Verification items for the finished model (mm, model axes). Face numbers are marked on the shaded views. A direction names the side the tool comes from. Round coordinates to 2 decimals unless told otherwise and drop trailing zeros. Write each loop counter-clockwise with the first axis right and the second up, starting at its lowest first coordinate (ties: lowest second). Pieces come first, ordered by that corner, then holes.
Autodesk Inventor part; units mm, degrees
ref_plane "YZ Plane" through (0, 0, 0) normal (1, 0, 0) x (0, 1, 0)
ref_plane "XZ Plane" through (0, 0, 0) normal (0, 1, 0) x (-1, 0, 0)
ref_plane "XY Plane" through (0, 0, 0) normal (0, 0, 1) x (1, 0, 0)
sketch "Block1" plane through (0, 0, 0) normal (0, 0, 1) x (1, 0, 0)
  circle A0 centre (74.029, 24.2723) radius 1
  line L0 (49.279, 30.4723) -> (71.779, 30.4723)
  line L1 (71.779, 30.4723) -> (71.779, 18.0723)
  line L2 (71.779, 18.0723) -> (49.279, 18.0723)
  line L3 (49.279, 18.0723) -> (49.279, 30.4723)
  line L4 (49.279, 30.4723) -> (44.779, 30.4723)
  line L5 (44.779, 30.4723) -> (44.779, 18.0723)
  line L6 (44.779, 18.0723) -> (49.279, 18.0723)
  line L7 (49.279, 18.0723) -> (49.279, 30.4723)
  line L8 (71.779, 30.4723) -> (76.279, 30.4723)
  line L9 (76.279, 30.4723) -> (76.279, 18.0723)
  line L10 (76.279, 18.0723) -> (71.779, 18.0723)
  line L11 (71.779, 18.0723) -> (71.779, 30.4723)
  line L12 (44.779, 24.2723) -> (76.279, 24.2723) construction
  line L13 (47.029, 30.4723) -> (47.029, 18.0723) construction
  circle A1 centre (47.029, 24.2723) radius 1
  line L14 (74.029, 30.4723) -> (74.029, 18.0723) construction
  point P0 (60.979, 24.0984)
  dimension "d7" = 22.5
  dimension "d8" = 12.4
  dimension "d9" = 4.5
  dimension "d10" = 4.5
  dimension "d11" = 2
  dimension "d12" = 2
sketch "Sketch1" plane through (0, 0, 0) normal (0, 0, 1) x (1, 0, 0)
  line L0 (-92.7646, -8.503) -> (-89.7646, -8.503)
  line L1 (-89.7646, -8.503) -> (-89.7646, -11.753)
  line L2 (-89.7646, -11.753) -> (-92.7646, -11.753)
  line L3 (-92.7646, -11.753) -> (-92.7646, -8.503)
  line L4 (-92.7646, -21.6527) -> (-89.7646, -21.6527)
  line L5 (-89.7646, -21.6527) -> (-89.7646, -21.7527)
  line L6 (-89.7646, -21.7527) -> (-92.7646, -21.7527)
  line L7 (-92.7646, -21.7527) -> (-92.7646, -21.6527)
  line L8 (-37.803, 27.4868) -> (-7.553, 27.4868)
  line L9 (-7.553, 27.4868) -> (-7.553, 9.4868)
  line L10 (-7.553, 9.4868) -> (-37.803, 9.4868)
  line L11 (-37.803, 9.4868) -> (-37.803, 27.4868)
  line L12 (-41.053, 25.4868) -> (-37.803, 25.4868)
  line L13 (-37.803, 25.4868) -> (-37.803, 11.4868)
  line L14 (-37.803, 11.4868) -> (-41.053, 11.4868)
  line L15 (-41.053, 11.4868) -> (-41.053, 25.4868)
  line L16 (-37.803, 18.4868) -> (-7.553, 18.4868) construction
  line L17 (-22.678, 27.4868) -> (-22.678, 9.4868) construction
  line L18 (-41.053, 18.4868) -> (-37.803, 18.4868) construction
  line L19 (-4.303, 25.4868) -> (-7.553, 25.4868)
  line L20 (-7.553, 25.4868) -> (-7.553, 11.4868)
  line L21 (-7.553, 11.4868) -> (-4.303, 11.4868)
  line L22 (-4.303, 11.4868) -> (-4.303, 25.4868)
  line L23 (-4.303, 18.4868) -> (-7.553, 18.4868) construction
  point P0 (0, 0)
  point P1 (-7.553, 18.4868)
  dimension "d0" = 3
  dimension "mat" = 3.25
  dimension "d2" = 3
  dimension "d3" = 0.1
  dimension "d38" = 30.25
  dimension "d39" = 18
  dimension "d40" = 3.25
  dimension "d41" = 14
extrude "Extrusion5" add sketch "Sketch1" along normal blind 3.25 contours L8 L9 L10 L11 | L11 L14 L15 L12 | L19 L22 L21 L9
equation "\"d40\" = mat"
equation "\"d42\" = mat"
properties part number "arm-servo"
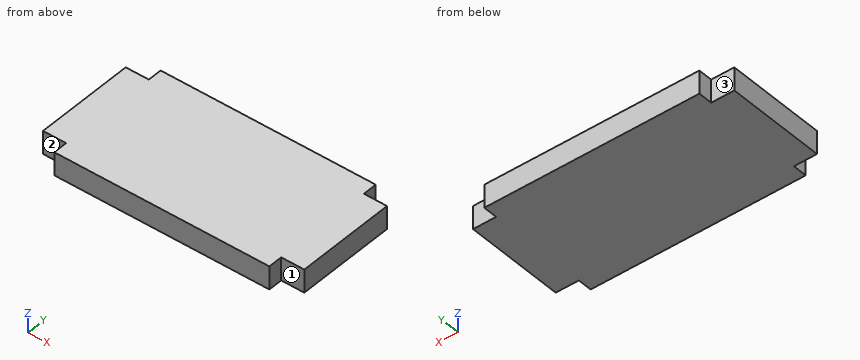
Q1. Sectioned sample at B-B (x = -7). Enter the section's corners in (y, z).
Recorded:
outline: (11.49, 0) - (25.49, 0) - (25.49, 3.25) - (11.49, 3.25) - close
Q2. Material ranges on line 1 along Y through (x, z) = (-6, 0.7), recorded low to high.
Recorded:
line 1: y = 11.49 to 25.49
Q3. Depth check by flat-ended pin: P1, Ø1.6, axis at x = -6.5, z = 1.5, coming from the +Y side; P2, Ø1, axis at x = -6, z = 2.5, coming from the -Y side; P3, Ø0.6, axis at y = 10.5, z = 2, coming from the +X side. Enter the tip coordinate at first touch or a pass-through.
Recorded:
P1: stops at y = 25.49
P2: stops at y = 11.49
P3: stops at x = -7.55
Q4. Tool access check on the marked faces 1, 2 and 3. Record the directions out of +Z, -Z, +X, -X, +Y, -Y that give a thin tool (end or side, any length) a straight path to the whole face; none if there is none.
Recorded:
face 1: +Z, -Z, +X, -Y
face 2: +Z, -Z, -X, -Y
face 3: +Z, -Z, -X, +Y
Q5. Sectioned sample at A-A (z = 0.5). Enter the section's corners in (x, y).
Recorded:
outline: (-41.05, 11.49) - (-37.8, 11.49) - (-37.8, 9.49) - (-7.55, 9.49) - (-7.55, 11.49) - (-4.3, 11.49) - (-4.3, 25.49) - (-7.55, 25.49) - (-7.55, 27.49) - (-37.8, 27.49) - (-37.8, 25.49) - (-41.05, 25.49) - close
